Read the model definition and answer for the solid it produces. Units are mm, in the model's axes. Face numbers are marked on the shaded views. A direction names the side the tool comes from. Give positions to 0.01 mm unless a question says otherwise; leave off trailing zeros. Order: outer loops, then holes, each group sorted by start corner. A loop starts at its lowest first (then second) coordinate and runs counter-clockwise, first axis right, second up. Notation, with made-up numbers: (18, 2.5) - (44, 2.5) arc R24 cw to (44, 41.5) - close; hole circle Ø11 at (88, -33). An arc over 180 degrees is marked (long way). Answer as CSV lines item,"result". Start each with the question number.
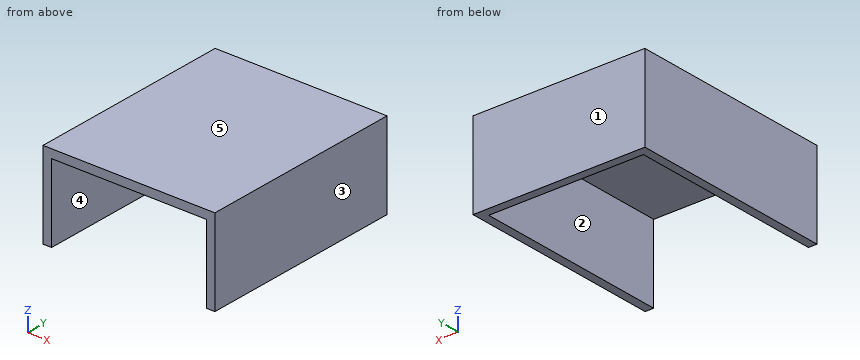
Autodesk Inventor part; units mm, degrees
ref_plane "YZ Plane" through (0, 0, 0) normal (1, 0, 0) x (0, 1, 0)
ref_plane "XZ Plane" through (0, 0, 0) normal (0, 1, 0) x (-1, 0, 0)
ref_plane "XY Plane" through (0, 0, 0) normal (0, 0, 1) x (1, 0, 0)
sketch "Sketch1" plane through (0, 0, 0) normal (0, 0, 1) x (1, 0, 0)
  line L0 (-50, 60) -> (50, 60)
  line L1 (50, 60) -> (50, -60)
  line L2 (50, -60) -> (-50, -60)
  line L3 (-50, -60) -> (-50, 60)
  point P0 (0, 0)
  dimension "d0" = 100
  dimension "d1" = 120
  dimension "d2" = 60
  dimension "d3" = 50
extrude "Extrusion1" add sketch "Sketch1" along normal mid plane 50
sketch "Sketch2" plane through (0, 0, -25) normal (0, 0, -1) x (-1, 0, 0)
  line L0 (-45, 55) -> (45, 55)
  line L1 (45, 55) -> (45, -60)
  line L2 (45, -60) -> (-45, -60)
  line L3 (-45, -60) -> (-45, 55)
  line L4 (-50, -60) -> (-50, 60)
  line L5 (-50, 60) -> (50, 60)
  line L6 (-50, 60) -> (50, 60)
  line L7 (50, -60) -> (-50, -60)
  line L8 (50, 60) -> (50, -60)
  line L9 (50, -60) -> (-50, -60)
  line L10 (-50, -60) -> (-50, 60)
  point P0 (0, 0)
  point P1 (0, -60)
  dimension "d6" = 5
  dimension "d7" = 5
  dimension "d8" = 5
extrude "Extrusion2" cut sketch "Sketch2" against normal blind 45 contours L0 L1 L2 L3
properties part number "casing"
(1) Straight lines are drawn through the part: line 1 (X direction, y = -2.5, z = -2); line 2 (Z direction, x = 43, y = 31); line 3 (Y direction, x = -35.5, z = 16). For each, find the intervals that lie inside material, in ascending order. Write a range as [from, to].
(2) Flat-ended cylindrical pins translate along their axes: pin 1 Ø3 at (x, z) = (-32.5, 6) entering from -Y; pin 2 Ø12 at (x, y) = (-14, 28.5) entering from -Z. Find the tip coordinate at first contact, or state that the pin passes through.
(3) Section A-A, the plane y = 36.5 is taken. Write down the section's boundary in (x, z).
(4) Determine the mould class of the marked faces 3, 4 and 5 for opening direction X: released by +X, released by -X, zero draft, split by the parting line, or undercut.
(5) Section B-B, the plane z = -2.5 is taken. Write down the section's boundary in (x, y).
(6) Which of the six approach directions +Z, -Z, +X, -X, +Y, -Y give full straight-line access (tool end or side, diameter ignored) to the marked faces 1 and 2?
(7) Section C-C, the plane x = 43.5 is taken. Write down the section's boundary in (y, z).
Checks:
1,line 1,"x = [-50, -45], [45, 50]"
1,line 2,"z = [20, 25]"
1,line 3,"y = [55, 60]"
2,pin 1,"stops at y = 55"
2,pin 2,"stops at z = 20"
3,outline,"(-50, -25) - (-45, -25) - (-45, 20) - (45, 20) - (45, -25) - (50, -25) - (50, 25) - (-50, 25) - close"
4,face 3,"released by +X"
4,face 4,"undercut"
4,face 5,"zero draft"
5,outline,"(-50, -60) - (-45, -60) - (-45, 55) - (45, 55) - (45, -60) - (50, -60) - (50, 60) - (-50, 60) - close"
6,face 1,"+Z, -Z, +X, -X, +Y"
6,face 2,"-Z, -Y"
7,outline,"(-60, 20) - (55, 20) - (55, -25) - (60, -25) - (60, 25) - (-60, 25) - close"
